The listing builds one solid part. Answer for the finished solid, in the listing's coordinates (mm). Coordinates: 2 decimals unless noted, no trailing zeros. Use a Markdown table: item, result. Add a question column.
Item 1: The mould has two halves that part along X. Classify faces 1 (the cylindrical face through (11.08, 70.12, -0.14)), 2 (the flat face through (0, -3, 0)), 3 (the flat face through (10, -3, 10)): released by +X, released by -X, zero draft, split by the parting line, or undercut.
Item 2: The part is cut by section A-A, the plane z = 5. State how many separate pieces and enclosed holes the cut face has, then the cut area to 3 significant figures.
Item 3: Find the intervals of material crossed by line 1 along X through (y, z) = (31, -4); line 2 along X through (y, z) = (185, 1.25), in increasing order.
from build123d import *

# Parameters (mm, degrees)
F0_W     = 400
F0_H     = 20
F1_DEPTH = 20
F3_D     = 5.5
F3_DEPTH = 20
F3_TIP   = 1.6523667023
F5_D     = 10
F5_DEPTH = 20
F5_TIP   = 3.0043030951
F7_DEPTH = 10


# Not quite as in the source:
# - a feature names something its author has since deleted; it is built from what else it names


with BuildPart() as f1:
    # F0 (on Right) → F1 (new body)
    with BuildSketch(Plane.YZ):
        Rectangle(F0_W, F0_H)
    extrude(amount=F1_DEPTH)

    # F3
    with Locations(Plane.XY.offset(10)):
        with Locations((10, 185), (10, 141), (10, 97), (10, -167), (10, -123), (10, -79), (10, -35), (10, 9), (10, 53)):
            Hole(F3_D / 2, depth=F3_DEPTH)
            with Locations((0, 0, -(F3_DEPTH + F3_TIP / 2))):  # 118° drill point
                Cone(0, F3_D / 2, F3_TIP, mode=Mode.SUBTRACT)

    # F5
    with Locations(Plane.XY.offset(10)):
        with Locations((10, 163), (10, 119), (10, 75), (10, -189), (10, -145), (10, -101), (10, -57), (10, -13), (10, 31)):
            Hole(F5_D / 2, depth=F5_DEPTH)
            with Locations((0, 0, -(F5_DEPTH + F5_TIP / 2))):  # 118° drill point
                Cone(0, F5_D / 2, F5_TIP, mode=Mode.SUBTRACT)

    # F6 (on face) → F7 (cut)
    with BuildSketch(Plane.YZ.offset(20)):
        with BuildLine():
            ThreePointArc((71, 10), (71.5, 9.5), (72, 10))
            Line((72, 10), (71, 10))
        make_face()
        with BuildLine():
            ThreePointArc((96.5, 10), (97, 9.5), (97.5, 10))
            Line((97.5, 10), (96.5, 10))
        make_face()
        with BuildLine():
            ThreePointArc((115, 10), (115.5, 9.5), (116, 10))
            Line((116, 10), (115, 10))
        make_face()
        with BuildLine():
            ThreePointArc((140.5, 10), (141, 9.5), (141.5, 10))
            Line((141.5, 10), (140.5, 10))
        make_face()
        with BuildLine():
            ThreePointArc((159, 10), (159.5, 9.5), (160, 10))
            Line((160, 10), (159, 10))
        make_face()
        with BuildLine():
            Line((185.5, 10), (184.5, 10))
            ThreePointArc((184.5, 10), (185, 9.5), (185.5, 10))
        make_face()
        with BuildLine():
            ThreePointArc((52.5, 10), (53, 9.5), (53.5, 10))
            Line((53.5, 10), (52.5, 10))
        make_face()
        with BuildLine():
            ThreePointArc((27, 10), (27.5, 9.5), (28, 10))
            Line((28, 10), (27, 10))
        make_face()
        with BuildLine():
            ThreePointArc((8.5, 10), (9, 9.5), (9.5, 10))
            Line((9.5, 10), (8.5, 10))
        make_face()
        with BuildLine():
            ThreePointArc((-17, 10), (-16.5, 9.5), (-16, 10))
            Line((-16, 10), (-17, 10))
        make_face()
        with BuildLine():
            ThreePointArc((-35.5, 10), (-35, 9.5), (-34.5, 10))
            Line((-34.5, 10), (-35.5, 10))
        make_face()
        with BuildLine():
            Line((-60, 10), (-61, 10))
            ThreePointArc((-61, 10), (-60.5, 9.5), (-60, 10))
        make_face()
        with BuildLine():
            Line((-78.5, 10), (-79.5, 10))
            ThreePointArc((-79.5, 10), (-79, 9.5), (-78.5, 10))
        make_face()
        with BuildLine():
            Line((-104, 10), (-105, 10))
            ThreePointArc((-105, 10), (-104.5, 9.5), (-104, 10))
        make_face()
        with BuildLine():
            Line((-122.5, 10), (-123.5, 10))
            ThreePointArc((-123.5, 10), (-123, 9.5), (-122.5, 10))
        make_face()
        with BuildLine():
            Line((-148, 10), (-149, 10))
            ThreePointArc((-149, 10), (-148.5, 9.5), (-148, 10))
        make_face()
        with BuildLine():
            Line((-166.5, 10), (-167.5, 10))
            ThreePointArc((-167.5, 10), (-167, 9.5), (-166.5, 10))
        make_face()
        with BuildLine():
            Line((-192, 10), (-193, 10))
            ThreePointArc((-193, 10), (-192.5, 9.5), (-192, 10))
        make_face()
    extrude(amount=-F7_DEPTH, mode=Mode.SUBTRACT)


solid = f1.part
Solution:
| question | item | result |
|---|---|---|
| 1 | face 1 | undercut |
| 1 | face 2 | released by -X |
| 1 | face 3 | zero draft |
| 2 | separate pieces | 1 |
| 2 | enclosed holes | 18 |
| 2 | area | 7,080 mm2 |
| 3 | line 1 | x = 0 to 5, 15 to 20 |
| 3 | line 2 | x = 0 to 7.25, 12.75 to 20 |
